Read the model definition and answer for the solid it produces. Units are mm, in the model's axes. Face numbers are marked on the shaded views. A direction names the side the tool comes from. Round coordinates to 2 decimals unless told otherwise and drop trailing zeros. Write each loop counter-clockwise with the first axis right and the second up, starting at its lowest first coordinate (ties: lowest second). Pieces come first, ordered by that corner, then holes. Notation, with made-up numbers: (-6, -9) - (9, -9) arc R20 ccw to (9, 1) - close; hole circle Ø9 at (65, 68.5). An arc over 180 degrees is marked (long way). One line per item, written item: value. Start each with the question number.
(1) Find the intervals of material crossed by L1, parallel to Y at x = -11, z = -2.5; L2, parallel to X at y = -4.5, z = 9.5, in increasing order.
(2) A cutting plane is placed at C-C, the plane y = -4.5. Determine the outline of the cut face in (x, z), plus the area to 3 significant figures.
(3) For the marked faces 1, 2 and 3, determine the directions among +Z, -Z, +X, -X, +Y, -Y from which every point of the face is accessible in a straight line to the end or side of a thin tool.
(4) A cutting plane is placed at D-D, the plane x = -17.5. Determine the outline of the cut face in (y, z), plus the area to 3 significant figures.
(5) A cutting plane is placed at A-A, the plane x = -2.5. Determine the outline of the cut face in (y, z).
(6) Flat-ended cylindrical pins translate along their axes: pin 1 Ø8 at (y, z) = (-6.5, 12.5) entering from +X; pin 2 Ø5 at (x, y) = (-1, -5) entering from -Z; pin 3 Ø2 at (x, z) = (-6, 23.5) entering from -Y. Find the tip coordinate at first contact, or state that the pin passes through.
(7) A cutting plane is placed at B-B, the plane z = 9. Determine the outline of the cut face in (x, y).
from build123d import *

# Parameters (mm, degrees)
F0_W     = 50
F0_H     = 40
F0_W_2   = 10
F0_H_2   = 10
F1_DEPTH = 40
F4_DEPTH = 10


with BuildPart() as f1:
    # F0 (on Front) → F1 (new body)
    with BuildSketch(Plane.XZ):
        with Locations((-0.869263, 12.341743)):
            Rectangle(F0_W, F0_H)
        with Locations((-0.869263, 12.341743)):
            Rectangle(F0_W_2, F0_H_2, mode=Mode.SUBTRACT)
        with Locations((-0.869263, 12.341743)):
            Rectangle(F0_W_2, F0_H_2)
    extrude(amount=-F1_DEPTH)

    # F0 (on Front) → F4 (join)
    with BuildSketch(Plane.XZ):
        with Locations((-0.869263, 12.341743)):
            Rectangle(F0_W_2, F0_H_2)
    extrude(amount=F4_DEPTH)


solid = f1.part
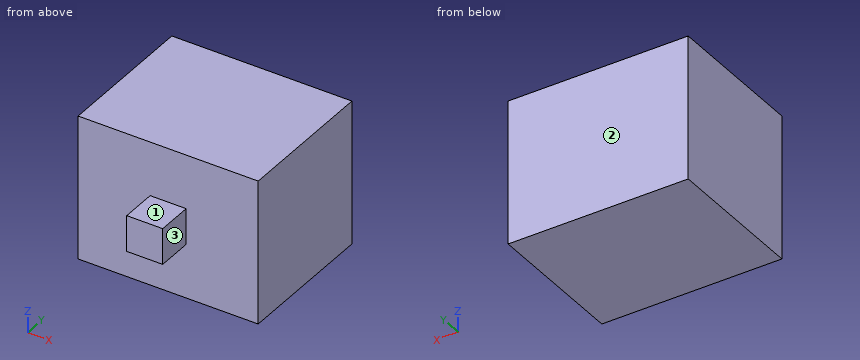
Here are the results:
1. L1: 0 to 40
1. L2: -5.87 to 4.13
2. outline: (-5.87, 7.34) - (4.13, 7.34) - (4.13, 17.34) - (-5.87, 17.34) - close
2. area: 100 mm²
3. face 1: +Z, +X, -X, -Y
3. face 2: +Z, -Z, +X, -X, +Y
3. face 3: +Z, -Z, +X, -Y
4. outline: (0, -7.66) - (40, -7.66) - (40, 32.34) - (0, 32.34) - close
4. area: 1,600 mm²
5. outline: (-10, 7.34) - (0, 7.34) - (0, -7.66) - (40, -7.66) - (40, 32.34) - (0, 32.34) - (0, 17.34) - (-10, 17.34) - close
6. pin 1: x = 4.13
6. pin 2: z = 7.34
6. pin 3: y = 0
7. outline: (-25.87, 0) - (-5.87, 0) - (-5.87, -10) - (4.13, -10) - (4.13, 0) - (24.13, 0) - (24.13, 40) - (-25.87, 40) - close
